Could you check a few things on this model? Use its own coordinates, in mm. Face numbers are marked on the shaded views. A direction names the side the tool comes from. Give positions to 0.01 mm unless a question says otherwise; leave off trailing zeros. Order: outer loops, then holes, each group sorted by start corner. A loop starts at its lowest first (then second) coordinate and runs counter-clockwise, first axis right, second up. Notation, with made-up numbers: M -35,-16.75 L -22,-16.75 A21 ccw -22,-0.75 Z; hole C -6,32.25 d2. An arc over 180 degrees is marked long. Answer in a Markdown table with one row per item. Add a question column.
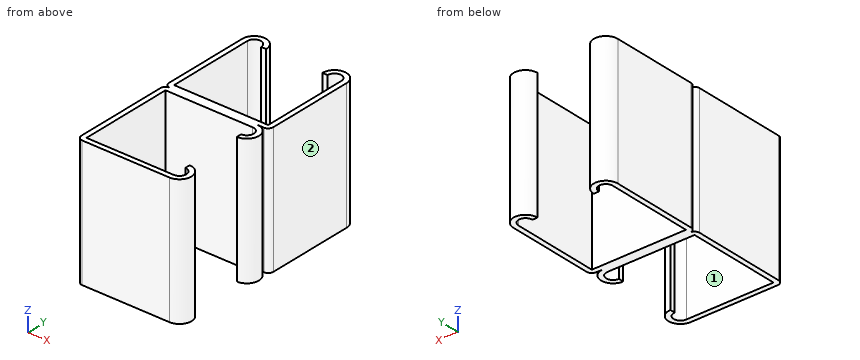
```python
from build123d import *

# Parameters (mm, degrees)
BASE_EXTRUDE_DEPTH = 12.7
CIRPATTERN1_COUNT  = 2
CIRPATTERN1_ANGLE  = 270


with BuildPart() as part:
    # Sketch1 → Base-Extrude (new, symmetric)
    with BuildSketch(Plane.XY):
        with BuildLine():
            Line((0, 18.25625), (0, 1.016))
            ThreePointArc((0, 1.016), (0.29757951, 0.29757951), (1.016, 0))
            Line((1.016, 0), (19.6215, 0))
            ThreePointArc((19.6215, 0), (20.33992049, 0.29757951), (20.6375, 1.016))
            Line((20.6375, 1.016), (20.6375, 18.25625))
            ThreePointArc((20.6375, 18.25625), (18.25625, 20.6375), (15.875, 18.25625))
            Line((15.875, 18.25625), (16.891, 18.25625))
            ThreePointArc((16.891, 18.25625), (18.25625, 19.6215), (19.6215, 18.25625))
            Line((19.6215, 18.25625), (19.6215, 1.016))
            Line((19.6215, 1.016), (1.016, 1.016))
            Line((1.016, 1.016), (1.016, 18.25625))
            ThreePointArc((1.016, 18.25625), (2.38125, 19.6215), (3.7465, 18.25625))
            Line((3.7465, 18.25625), (4.7625, 18.25625))
            ThreePointArc((4.7625, 18.25625), (2.38125, 20.6375), (0, 18.25625))
        make_face()
    base_extrude = extrude(amount=BASE_EXTRUDE_DEPTH, both=True)

    # CirPattern1: Base-Extrude ×2 about axis
    cirpattern1_axis = Axis((0, 0, 0), (0, 0, 1))
    for i in range(1, CIRPATTERN1_COUNT):
        add(base_extrude.rotate(cirpattern1_axis, i * CIRPATTERN1_ANGLE / (CIRPATTERN1_COUNT - 1)))


solid = part.part
```
1. For the marked faces 1 and 2, which set-ups out of +Z, -Z, +X, -X, +Y, -Y let a thin tool reach every point of the face, with its end or its side?
2. Suppose I cut it at D-D on x = 2. List the corners of the cut face in (y, z) for me, plus the area to 3 significant figures.
3. If I drill on line 1 along Y through (x, z) = (7.25, -3.75); line 2 along X through (y, z) = (-2.5, 3.5); line 3 along Y through (x, z) = (4.5, 2.5), over which ranges is the centre line in solid material (lowest first)? Write a range as [from, to].
4. Suppose I cut it at A-A on x = 15. List the corners of the cut face in (y, z) for me, plus the area to 3 significant figures.
5. Suppose I cut it at C-C on z = 1. List the corners of the cut face in (x, y) for me (1 decimal).
6. Will these pins go through, and if not, where does the flat tip stop? P1, Ø15, axis at y = -10, z = -6, coming from the +X side; P2, Ø9.5, axis at x = 8, z = 3, coming from the +Y side; P3, Ø5, axis at x = 10, z = 5.5, coming from the +Y side.
7. Suppose I cut it at B-B on y = 9. List the corners of the cut face in (x, z) for me, plus the area to 3 significant figures.
Findings below:
| question | item | result |
|---|---|---|
| 1 | face 1 | +Z, -Z |
| 1 | face 2 | +Z, -Z, +X, +Y, -Y |
| 2 | outline | M -20.64,-12.7 L -19.62,-12.7 L -19.62,12.7 L -20.64,12.7 Z; M -1.02,-12.7 L 1.02,-12.7 L 1.02,12.7 L -1.02,12.7 Z; M 19.57,-12.7 L 20.61,-12.7 L 20.61,12.7 L 19.57,12.7 Z |
| 2 | area | 104 mm2 |
| 3 | line 1 | [-20.64, -19.62], [-1.02, 1.02] |
| 3 | line 2 | [0, 1.02], [19.62, 20.63] |
| 3 | line 3 | [-20.64, -19.62], [-1.02, 1.02], [18.26, 19.34] |
| 4 | outline | M -20.64,-12.7 L -19.62,-12.7 L -19.62,12.7 L -20.64,12.7 Z; M -1.02,-12.7 L 1.02,-12.7 L 1.02,12.7 L -1.02,12.7 Z |
| 4 | area | 77.4 mm2 |
| 5 | outline | M 0,-19.6 A1 ccw 1,-20.6 L 18.3,-20.6 A2.4 ccw 18.3,-15.9 L 18.3,-16.9 A1.4 cw 18.3,-19.6 L 1,-19.6 L 1,-1 L 18.3,-1 A1.4 cw 18.3,-3.7 L 18.3,-4.8 A2.4 ccw 18.3,0 L 19.6,0 A1 ccw 20.6,1 L 20.6,18.3 A2.4 ccw 15.9,18.3 L 16.9,18.3 A1.4 cw 19.6,18.3 L 19.6,1 L 1,1 L 1,18.3 A1.4 cw 3.7,18.3 L 4.8,18.3 A2.4 ccw 0,18.3 L 0,1 A1 ccw 1,0 A1 ccw 0,-1 Z |
| 6 | P1 | x = 20.63 |
| 6 | P2 | y = 20.47 |
| 6 | P3 | y = 1.02 |
| 7 | outline | M 0,-12.7 L 1.02,-12.7 L 1.02,12.7 L 0,12.7 Z; M 19.62,-12.7 L 20.64,-12.7 L 20.64,12.7 L 19.62,12.7 Z |
| 7 | area | 51.6 mm2 |
